For this review, take the finished solid that the model builds, in its own axes (mm). A direction names the side the tool comes from. Round coordinates to 2 decimals unless told otherwise and drop trailing zeros. Order: outer loops, then holes, each group sorted by start corner. A loop starts at its lowest first (then second) coordinate and runs counter-clockwise, first axis right, second up. Notation, with made-up numbers: (64.5, -30.75) - (89.5, -30.75) arc R27 cw to (89.5, -2.75) - close; hole circle Ø1 at (-26, 31.25). An arc over 180 degrees is marked (long way). Write each question's results on one line, items separated by ' | '. Start each with the question number.
(1) Take a section at B-B, the plane x = -5.5. Give the boundary of the cut face in (y, z).
(2) Insertion check: pin 1 Ø1 at (x, z) = (14, 14.5) entering from +Y; pin 2 Ø3 at (y, z) = (21.5, 48) entering from -X; pin 3 Ø5.5 at (x, y) = (-2, -3.5) entering from +Z. Each pin has a flat end and moves straight along its axis. Give the tip position at first contact, or say it passes through.
(3) Take a section at A-A, the plane z = 82.5. Give the number of separate pieces and of enclosed holes in the cut face, plus the area to 3 significant figures.
(4) For faces 1 (the flat face through (0, 0, 73)), 2 (the cylindrical face through (16.794, 25.434, 34.51)), 3 (the flat face through (17, 2, 70)), list the 3-axis set-ups (+Z, -Z, +X, -X, +Y, -Y) from which the entire face can be reached by the end or side of a thin tool; tool diameter is ignored.
(5) Draft analysis for pull direction X (two halves, no side actions). For faces 4 (the conical face through (12.57, -21.11, 71.29)), 5 (the conical face through (-12.57, 21.11, 71.29)), 6 (the cylindrical face through (16.169, 8.526, 79.914)), state which applies: pulls with the +X half, pulls with the -X half, needs draft (parallel to the pull), parting line crosses it, or undercut.
(6) For L1, parallel to Z at x = 17, y = -18.5; L2, parallel to Z at x = -9, y = -10; L3, parallel to X at y = 19.5, z = 16.5, list the stretches that pass through material, from the lowest coordinate up. Write a range as from..to.
(7) Take a section at C-C, the plane z = 26. Give the boundary of the cut face in (x, y), plus the area to 3 significant figures.
```python
from build123d import *

# Parameters (mm, degrees)
BOSS_EXTRUDE1_DEPTH = 70
BOSS_EXTRUDE2_DEPTH = 3
BOSS_EXTRUDE2_TAPER = 67
SKETCH3_R           = 1.75
SKETCH3_R_2         = 0.75
BOSS_EXTRUDE3_DEPTH = 20


with BuildPart() as part:
    # Sketch1 → Boss-Extrude1 (new body)
    with BuildSketch(Plane(origin=(0, 0, 0), x_dir=(0, 1, 0), z_dir=(0, 0, 1))):
        with BuildLine():
            Line((-19, 19.5), (19, 19.5))
            ThreePointArc((19, 19.5), (25.363961031, 16.863961031), (28, 10.5))
            Line((28, 10.5), (28, -10.5))
            ThreePointArc((28, -10.5), (25.363961031, -16.863961031), (19, -19.5))
            Line((19, -19.5), (-19, -19.5))
            ThreePointArc((-19, -19.5), (-25.363961031, -16.863961031), (-28, -10.5))
            Line((-28, -10.5), (-28, 10.5))
            ThreePointArc((-28, 10.5), (-25.363961031, 16.863961031), (-19, 19.5))
        make_face()
    extrude(amount=BOSS_EXTRUDE1_DEPTH)

    # Sketch2 → Boss-Extrude2 (add)
    with BuildSketch(Plane.XY.offset(70)):
        with BuildLine():
            Line((10.5, 25), (-10.5, 25))
            ThreePointArc((-10.5, 25), (-14.742640687, 23.242640687), (-16.5, 19))
            Line((-16.5, 19), (-16.5, -19))
            ThreePointArc((-16.5, -19), (-14.742640687, -23.242640687), (-10.5, -25))
            Line((-10.5, -25), (10.5, -25))
            ThreePointArc((10.5, -25), (14.742640687, -23.242640687), (16.5, -19))
            Line((16.5, -19), (16.5, 19))
            ThreePointArc((16.5, 19), (14.742640687, 23.242640687), (10.5, 25))
        make_face()
    extrude(amount=BOSS_EXTRUDE2_DEPTH, taper=BOSS_EXTRUDE2_TAPER)

    # Sketch3 → Boss-Extrude3 (add)
    with BuildSketch(Plane.XY.offset(70)):
        with Locations((14.5, 8)):
            Circle(SKETCH3_R)
        with Locations((14.5, 4)):
            Circle(SKETCH3_R)
        with Locations(Location((-16.5, 18, 0), (0, 0, 270))):
            Circle(SKETCH3_R_2)
        with Locations(Location((-16.5, 16.4, 0), (0, 0, 270))):
            Circle(SKETCH3_R_2)
        with Locations(Location((-16.5, 14.8, 0), (0, 0, 270))):
            Circle(SKETCH3_R_2)
        with Locations(Location((-16.5, 13.2, 0), (0, 0, 270))):
            Circle(SKETCH3_R_2)
        with Locations(Location((-16.5, 11.6, 0), (0, 0, 270))):
            Circle(SKETCH3_R_2)
        with Locations(Location((-16.5, 10, 0), (0, 0, 270))):
            Circle(SKETCH3_R_2)
        with Locations(Location((-16.5, 8.4, 0), (0, 0, 270))):
            Circle(SKETCH3_R_2)
    extrude(amount=BOSS_EXTRUDE3_DEPTH)


solid = part.part
```
Results below:
1) outline: (-28, 0) - (28, 0) - (28, 70) - (25, 70) - (17.93, 73) - (-17.93, 73) - (-25, 70) - (-28, 70) - close
2) pin 1: stops at y = 27.49 | pin 2: stops at x = -19.44 | pin 3: stops at z = 73
3) separate pieces: 9 | enclosed holes: 0 | area: 31.6 mm^2
4) face 1: +Z, +Y, -Y | face 2: +Z, -Z, +X, +Y | face 3: +Z
5) face 4: pulls with the +X half | face 5: pulls with the -X half | face 6: undercut
6) L1: z = 0..70 | L2: z = 0..73 | L3: x = -19.49..19.49
7) outline: (-19.5, -19) arc R9 ccw to (-10.5, -28) - (10.5, -28) arc R9 ccw to (19.5, -19) - (19.5, 19) arc R9 ccw to (10.5, 28) - (-10.5, 28) arc R9 ccw to (-19.5, 19) - close | area: 2,110 mm^2
